from build123d import *

# Parameters (mm, degrees)
SKETCH_1_W      = 55
SKETCH_1_H      = 60
SKETCH_1_W_2    = 36
SKETCH_1_H_2    = 40
EXTRUDE_1_DEPTH = 14
SKETCH_2_R      = 4
EXTRUDE_2_DEPTH = 60


with BuildPart() as part:
    # 草图1 → 凸台-拉伸1 (new body)
    with BuildSketch(Plane(origin=(0, 0, 0), x_dir=(1, 0, 0), z_dir=(0, 1, 0))):
        with Locations((27.5, 30)):
            Rectangle(SKETCH_1_W, SKETCH_1_H)
        with Locations((27, 30)):
            Rectangle(SKETCH_1_W_2, SKETCH_1_H_2, mode=Mode.SUBTRACT)
    extrude(amount=EXTRUDE_1_DEPTH)

    # 草图2 → 凸台-拉伸2 (add)
    with BuildSketch(Plane.XY):
        with BuildLine():
            Line((0, 0), (-20, 0))
            ThreePointArc((-20, 0), (-27, 7), (-20, 14))
            Line((-20, 14), (0, 14))
            Line((0, 14), (0, 0))
        make_face()
        with Locations((-20, 7)):
            Circle(SKETCH_2_R, mode=Mode.SUBTRACT)
    extrude(amount=-EXTRUDE_2_DEPTH)


solid = part.part
Part model, mm, in its own coordinate system. A direction names the side the tool comes from. Give positions to 0.01 mm unless a question says otherwise; leave off trailing zeros. Loops run counter-clockwise (first coordinate to the right, second up) from the corner with the lowest first, then second, coordinate; pieces in that order, holes last.
(1) 3-axis set-ups, long thin cutter, end or side, ignore diameter. For faces 4 (the flat face through (9, 7, -30)), 5 (the cylindrical face through (-23.2, 4.6, -29.6)): which of +Z, -Z, +X, -X, +Y, -Y reach the whole face in a straight line?
Return value:
face 4: +Y, -Y
face 5: +Z, -Z
(2) Pin check, flat tip, straight feed: pin 1 (7 mm diameter, centred on y = 5, z = -38.5, fed in from -X). Stop position of the tip, or through.
Return value:
pin 1: stops at x = -27
(3) Drill centre lines: line 1 along Z through (x, y) = (37, 7.75); line 2 along Y through (x, z) = (-20, -24); line 3 along X through (y, z) = (9, -45.5). Where is each one in solid material? Low to high.
Return value:
line 1: z = -60 to -50, -10 to 0
line 2: y = 0 to 3, 11 to 14
line 3: x = -26.71 to -23.46, -16.54 to 9, 45 to 55
(4) Band-saw the part on C-C (x = 37.5). Write the cut outline in (y, z), and give its area (3 significant figures).
Return value:
outline: (0, -60) - (14, -60) - (14, -50) - (0, -50) - close; (0, -10) - (14, -10) - (14, 0) - (0, 0) - close
area: 280 mm2
(5) Band-saw the part on D-D (y = 2). Write the cut outline in (x, z), and give its area (3 significant figures).
Return value:
outline: (-24.9, -60) - (55, -60) - (55, 0) - (-24.9, 0) - close; hole (9, -50) - (45, -50) - (45, -10) - (9, -10) - close
area: 3,350 mm2
(6) Pull direction Z, two halves, no side cores. Call faces 1 (the flat face through (45, 7, -30)), 2 (the flat face through (8.6, 14, -29.6)), 3 (the flat face through (15, 7, 0)): pulls with the +Z half, pulls with the -Z half, needs draft (parallel to the pull), parting line crosses it, or undercut.
Return value:
face 1: undercut
face 2: needs draft
face 3: pulls with the +Z half
(7) Band-saw the part on A-A (z = -11). Write the cut outline in (x, y).
Return value:
outline: (-20, 0) - (9, 0) - (9, 14) - (-20, 14) arc R7 ccw to start; (45, 0) - (55, 0) - (55, 14) - (45, 14) - close; hole circle Ø8 at (-20, 7)
(8) Band-saw the part on B-B (y = 7). Write the cut outline in (x, z), and give its area (3 significant figures).
Return value:
outline: (-27, -60) - (-24, -60) - (-24, 0) - (-27, 0) - close; (-16, -60) - (55, -60) - (55, 0) - (-16, 0) - close; hole (9, -50) - (45, -50) - (45, -10) - (9, -10) - close
area: 3,000 mm2
